Verification items for the finished model (mm, model axes). Face numbers are marked on the shaded views. A direction names the side the tool comes from. Coordinates: 2 decimals unless noted, no trailing zeros. Order: outer loops, then holes, each group sorted by start corner. A loop starts at its lowest first (then second) coordinate and runs counter-clockwise, first axis right, second up. Notation, with made-up numbers: (-36.5, 1.5) -> (-30.5, 1.5) arc R13 cw to (-30.5, 18.5) -> close; hole circle Ø4 at (36.5, 40.5). An arc over 180 degrees is marked (long way). Answer as CSV lines item,"result".
```python
from build123d import *

# Parameters (mm, degrees)
SALIENTE_EXTRUIR1_DEPTH      = 3.5
CROQUIS2_R                   = 2.5
CORTAR_EXTRUIR1_DEPTH        = 7.25
CORTAR_EXTRUIR1_DEPTH_BACK   = 13.5
TALADRO_DE_MARGEN_PARA_M31_D = 3.4
CHAFL_N1_SIZE                = 3
CHAFL_N2_SIZE                = 0.5
CHAFL_N3_SIZE                = 0.5


with BuildPart() as part:
    # Croquis1 → Saliente-Extruir1 (new body, symmetric)
    with BuildSketch(Plane.XY):
        Polygon((6.25, 60), (6.25, 65), (0, 65), (-12.5, 65), (-12.5, 3.5), (-12.5, -3.5), (-2.5, -3.5), (-2.5, 3.5), (-7.5, 3.5), (-7.5, 60), (0, 60), align=None)
    extrude(amount=SALIENTE_EXTRUIR1_DEPTH, both=True)

    # Croquis2 → Cortar-Extruir1 (cut, two sides)
    with BuildSketch(Plane(origin=(0, 0, 0), x_dir=(0, 0, -1), z_dir=(1, 0, 0))) as cortar_extruir1_sk:
        Circle(CROQUIS2_R)
    extrude(amount=CORTAR_EXTRUIR1_DEPTH, mode=Mode.SUBTRACT)
    extrude(cortar_extruir1_sk.sketch, amount=-CORTAR_EXTRUIR1_DEPTH_BACK, mode=Mode.SUBTRACT)

    # Taladro de margen para M31 (through all)
    with Locations(Plane(origin=(0, 65, 0), x_dir=(1, 0, 0), z_dir=(0, 1, 0))):
        with Locations((0, 0)):
            Hole(TALADRO_DE_MARGEN_PARA_M31_D / 2)

    # Chaflán1
    chafl_n1_edges = [part.edges().sort_by_distance(p)[0] for p in [
        (-7.5, 60, 0),
        (-7.5, 3.5, 0),
        (-12.5, 65, 0),
    ]]
    chamfer(chafl_n1_edges, length=CHAFL_N1_SIZE)

    # Chaflán2
    chafl_n2_edges = [part.edges().sort_by_distance(p)[0] for p in [
        (-3.5, 3.5, -3.5),
        (-2.5, 0, -3.5),
        (-7.5, -3.5, -3.5),
        (6.25, 62.5, 3.5),
        (-12.5, 29.25, -3.5),
        (6.25, 62.5, -3.5),
        (-12.5, 29.25, 3.5),
        (-7.5, -3.5, 3.5),
        (-2.5, 0, 3.5),
        (-3.5, 3.5, 3.5),
        (-7.5, 31.75, -3.5),
        (-7.5, 31.75, 3.5),
        (0.875, 60, -3.5),
        (-1.625, 65, -3.5),
        (-11, 63.5, -3.5),
        (-1.625, 65, 3.5),
        (0.875, 60, 3.5),
        (-11, 63.5, 3.5),
        (-6, 5, -3.5),
        (-6, 5, 3.5),
        (-6, 58.5, -3.5),
        (-6, 58.5, 3.5),
    ]]
    chamfer(chafl_n2_edges, length=CHAFL_N2_SIZE)

    # Chaflán3
    chafl_n3_edges = [part.edges().sort_by_distance(p)[0] for p in [
        (-2.5, -3.5, 0),
        (-12.5, -3.5, 0),
        (-2.5, 3.5, 0),
        (6.25, 60, 0),
        (6.25, 65, 0),
    ]]
    chamfer(chafl_n3_edges, length=CHAFL_N3_SIZE)


solid = part.part
```
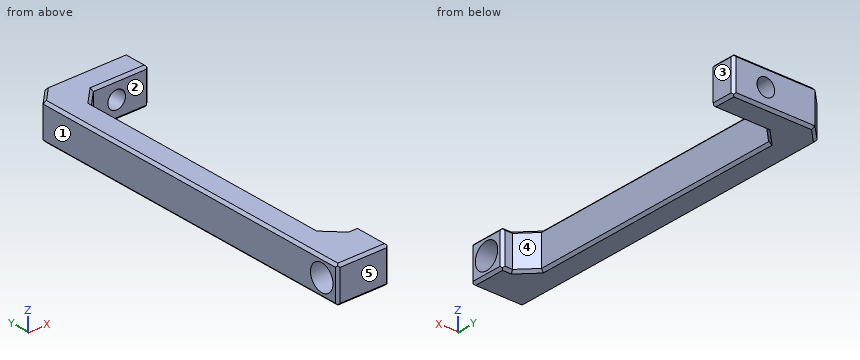
Item 1: Thickness scan on line 1 (Y direction, x = -4.5, z = 1); line 2 (Z direction, x = 0, y = 61.8); line 3 (Y direction, x = -8, z = 0). Record the ranges inside material, lowest first.
Answer list:
line 1,"-3.5 to -2.29, 2.29 to 3.5, 60 to 65"
line 2,"-3.5 to -1.7, 1.7 to 3.5"
line 3,"-3.5 to -2.5, 2.5 to 65"
Item 2: Section check D-D, the plane y = 41. Record the boundary of the cut face in (x, z).
Answer list:
outline,"(-12.5, -3) -> (-12, -3.5) -> (-8, -3.5) -> (-7.5, -3) -> (-7.5, 3) -> (-8, 3.5) -> (-12, 3.5) -> (-12.5, 3) -> close"
Item 3: Tool access check on the marked faces 1 and 2. Record the directions out of +Z, -Z, +X, -X, +Y, -Y that give a thin tool (end or side, any length) a straight path to the whole face; none if there is none.
Answer list:
face 1,"+Z, -Z, -X, +Y, -Y"
face 2,"+Z, -Z, +X"
Item 4: Section check B-B, the plane z = 0. Record the boundary of the cut face in (x, y).
Answer list:
outline,"(-12.5, -3) -> (-12, -3.5) -> (-3, -3.5) -> (-2.5, -3) -> (-2.5, -2.5) -> (-12.5, -2.5) -> close; (-12.5, 2.5) -> (-2.5, 2.5) -> (-2.5, 3) -> (-3, 3.5) -> (-4.5, 3.5) -> (-7.5, 6.5) -> (-7.5, 57) -> (-4.5, 60) -> (-1.7, 60) -> (-1.7, 65) -> (-9.5, 65) -> (-12.5, 62) -> close; (1.7, 60) -> (5.75, 60) -> (6.25, 60.5) -> (6.25, 64.5) -> (5.75, 65) -> (1.7, 65) -> close"
Item 5: Section check A-A, the plane x = 0. Record the boundary of the cut face in (y, z), plus the area to 3 significant figures.
Answer list:
outline,"(60, -3) -> (60.5, -3.5) -> (64.5, -3.5) -> (65, -3) -> (65, -1.7) -> (60, -1.7) -> close; (60, 1.7) -> (65, 1.7) -> (65, 3) -> (64.5, 3.5) -> (60.5, 3.5) -> (60, 3) -> close"
area,"17.5 mm2"
Item 6: Section check C-C, the plane y = 0. Record the boundary of the cut face in (x, z), plus the area to 3 significant figures.
Answer list:
outline,"(-12.5, -3) -> (-12, -3.5) -> (-3, -3.5) -> (-2.5, -3) -> (-2.5, -2.5) -> (-12.5, -2.5) -> close; (-12.5, 2.5) -> (-2.5, 2.5) -> (-2.5, 3) -> (-3, 3.5) -> (-12, 3.5) -> (-12.5, 3) -> close"
area,"19.5 mm2"
Item 7: Depth check by flat-ended pin: pin 1 Ø1.5 at (x, z) = (3, 0.5) entering from -Y; pin 2 Ø3 at (y, z) = (26, -2) entering from +X; pin 3 Ø8 at (x, y) = (0, 51) entering from +Z; pin 4 Ø5 at (x, y) = (-7.5, 31.5) entering from +Z. Enter the tip coordinate at first touch or a pass-through.
Answer list:
pin 1,"y = 60"
pin 2,"x = -7.5"
pin 3,"through"
pin 4,"z = 3.5"
Item 8: Release check for a two-part mould opening along Y. For the marked faces 3, 4 and 5 record: +Y half, -Y half, draft (parallel to the pull), parting line (faces both ways), or undercut.
Answer list:
face 3,"draft"
face 4,"undercut"
face 5,"-Y half"
